Could you check a few things on this model? Use its own coordinates, in mm. A direction names the side the tool comes from. Give positions to 0.01 mm unless a question says otherwise; leave off trailing zeros. Order: outer loops, then holes, each group sorted by start corner. A loop starts at its lowest first (then second) coordinate and runs counter-clockwise, first axis right, second up.
from build123d import *

# Parameters (mm, degrees)
BOSS_EXTRUDE1_DEPTH = 175
CUT_EXTRUDE1_DEPTH  = 176
CUT_EXTRUDE2_DEPTH  = 176
BOSS_EXTRUDE2_DEPTH = 125
CUT_EXTRUDE3_DEPTH  = 110
BOSS_EXTRUDE3_DEPTH = 65
CUT_EXTRUDE4_DEPTH  = 50
SKETCH3_W           = 200
SKETCH3_H           = 45
BOSS_EXTRUDE4_DEPTH = 15


with BuildPart() as part:
    # Sketch1 → Boss-Extrude1 (new body)
    with BuildSketch(Plane.XY):
        Polygon((-75, -12.5), (-100, -12.5), (-100, -62.5), (100, -62.5), (100, -12.5), (75, -12.5), align=None)
        Polygon((-25, 37.5), (-75, -12.5), (75, -12.5), (25, 37.5), align=None)
        Polygon((0, 62.5), (-25, 37.5), (25, 37.5), align=None)
        Polygon((25, 37.5), (75, -12.5), (100, -12.5), (100, 37.5), align=None)
        Polygon((0, 62.5), (25, 37.5), (100, 37.5), (100, 62.5), align=None)
        Polygon((-100, 62.5), (-100, 37.5), (-25, 37.5), (0, 62.5), align=None)
        Polygon((-100, 37.5), (-100, -12.5), (-75, -12.5), (-25, 37.5), align=None)
    extrude(amount=BOSS_EXTRUDE1_DEPTH)

    # Sketch1_3 → Cut-Extrude1 (cut, through all)
    with BuildSketch(Plane.XY):
        Polygon((0, 62.5), (25, 37.5), (100, 37.5), (100, 62.5), align=None)
        Polygon((-100, 62.5), (-100, 37.5), (-25, 37.5), (0, 62.5), align=None)
    extrude(amount=CUT_EXTRUDE1_DEPTH, mode=Mode.SUBTRACT)

    # Sketch1_4 → Cut-Extrude2 (cut, through all)
    with BuildSketch(Plane.XY):
        Polygon((-100, 37.5), (-100, -12.5), (-75, -12.5), (-25, 37.5), align=None)
        Polygon((25, 37.5), (75, -12.5), (100, -12.5), (100, 37.5), align=None)
    extrude(amount=CUT_EXTRUDE2_DEPTH, mode=Mode.SUBTRACT)

    # Sketch1_5 → Boss-Extrude2 (add)
    with BuildSketch(Plane.XY):
        Polygon((-100, 37.5), (-100, -12.5), (-75, -12.5), (-25, 37.5), align=None)
        Polygon((25, 37.5), (75, -12.5), (100, -12.5), (100, 37.5), align=None)
    extrude(amount=BOSS_EXTRUDE2_DEPTH)

    # Sketch1_6 → Cut-Extrude3 (cut)
    with BuildSketch(Plane.XY):
        Polygon((-100, 37.5), (-100, -12.5), (-75, -12.5), (-25, 37.5), align=None)
        Polygon((25, 37.5), (75, -12.5), (100, -12.5), (100, 37.5), align=None)
    extrude(amount=CUT_EXTRUDE3_DEPTH, mode=Mode.SUBTRACT)

    # Sketch1_9 → Boss-Extrude3 (add)
    with BuildSketch(Plane.XY):
        Polygon((25, 37.5), (75, -12.5), (100, -12.5), (100, 37.5), align=None)
        Polygon((-100, 37.5), (-100, -12.5), (-75, -12.5), (-25, 37.5), align=None)
    extrude(amount=BOSS_EXTRUDE3_DEPTH)

    # Sketch1_10 → Cut-Extrude4 (cut)
    with BuildSketch(Plane.XY):
        Polygon((25, 37.5), (75, -12.5), (100, -12.5), (100, 37.5), align=None)
        Polygon((-100, 37.5), (-100, -12.5), (-75, -12.5), (-25, 37.5), align=None)
    extrude(amount=CUT_EXTRUDE4_DEPTH, mode=Mode.SUBTRACT)

    # Sketch3 → Boss-Extrude4 (add)
    with BuildSketch(Plane(origin=(0, -12.5, 0), x_dir=(1, 0, 0), z_dir=(0, 1, 0))):
        with Locations((0, -87.5)):
            Rectangle(SKETCH3_W, SKETCH3_H)
    extrude(amount=BOSS_EXTRUDE4_DEPTH)


solid = part.part
Item 1: For faces 1 (the flat face through (-71, 18, 50)), 2 (the flat face through (80, 2.5, 87)), 3 (the flat face through (87, -12.5, 25)), 4 (the flat face through (-88, -12.5, 150)), which set-ups out of +Z, -Z, +X, -X, +Y, -Y let a thin tool reach every point of the face, with its end or its side?
Findings:
face 1: -Z, -X, +Y
face 2: +X, +Y
face 3: -Z, +X, +Y
face 4: +Z, -X, +Y
Item 2: Imagine slicing it at A-A on y = 18.5. List the corners of the cut face in (x, z) for me, then the cut area to 3 significant figures.
Findings:
outline: (-100, 50) - (-44, 50) - (-44, 0) - (44, 0) - (44, 50) - (100, 50) - (100, 65) - (44, 65) - (44, 110) - (100, 110) - (100, 125) - (44, 125) - (44, 175) - (-44, 175) - (-44, 125) - (-100, 125) - (-100, 110) - (-44, 110) - (-44, 65) - (-100, 65) - close
area: 18,800 mm2
Item 3: We'd pull the mould along Z, two halves only. Please class faces 5 (the flat face through (70, 18, 50)), 6 (the flat face through (-38, 24.5, 86.3)), 7 (the flat face through (63, 37.5, 57)), 8 (the flat face through (70, 20, 110)): +Z half, -Z half, draft (parallel to the pull), parting line (faces both ways), or undercut.
Findings:
face 5: -Z half
face 6: undercut
face 7: draft
face 8: undercut
Item 4: Imagine slicing it at B-B on z = 164. List the corners of the cut face in (x, y) for me.
Findings:
outline: (-100, -62.5) - (100, -62.5) - (100, -12.5) - (75, -12.5) - (0, 62.5) - (-75, -12.5) - (-100, -12.5) - close
Item 5: Imagine slicing it at D-D on y = -6.5. List the corners of the cut face in (x, z) for me, then the cut area to 3 significant figures.
Findings:
outline: (-100, 50) - (-69, 50) - (-69, 0) - (69, 0) - (69, 50) - (100, 50) - (100, 125) - (69, 125) - (69, 175) - (-69, 175) - (-69, 125) - (-100, 125) - close
area: 28,800 mm2
Item 6: For pin 1 (12.5 mm diameter, centred on x = 92.5, z = 35, fed in from +Y); pin 2 (15 mm diameter, centred on x = 53.5, y = 24, fed in from +Z); pin 3 (4 mm diameter, centred on y = 17.5, z = 105, fed in from +X), each with a flat end and sliding along its axis, tell me the tip position at first contact or that it passes through.
Findings:
pin 1: stops at y = -12.5
pin 2: stops at z = 125
pin 3: stops at x = 47
Item 7: Imagine slicing it at C-C on x = -50.5. List the corners of the cut face in (y, z) for me.
Findings:
outline: (-62.5, 0) - (12, 0) - (12, 50) - (37.5, 50) - (37.5, 65) - (12, 65) - (12, 110) - (37.5, 110) - (37.5, 125) - (12, 125) - (12, 175) - (-62.5, 175) - close
Item 8: Please list where these lines run through material, in increasing order: line 1 along Z through (x, y) = (-52, 29); line 2 along Y through (x, z) = (87, 28); line 3 along Y through (x, z) = (72, 80).
Findings:
line 1: z = 50 to 65, 110 to 125
line 2: y = -62.5 to -12.5
line 3: y = -62.5 to 2.5
